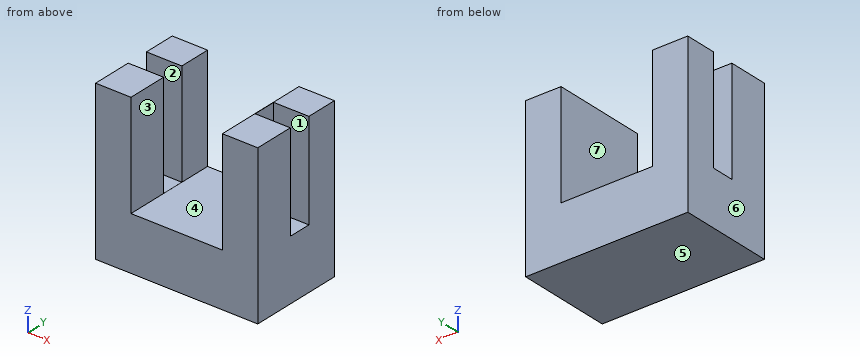
```python
from build123d import *

# Parameters (mm, degrees)
F1_DEPTH = 33.782
F2_DEPTH = 1.016
F3_W     = 12.5559801236
F3_H     = 8.0651557073
F4_DEPTH = 37.0078
F3_W_2   = 12.5338770449
F3_H_2   = 8.1778438762
F5_DEPTH = 34.544


with BuildPart() as f1:
    # F0 (on Front) → F1 (new body)
    with BuildSketch(Plane.XZ):
        Polygon((0, 56.0894832015), (0, 0), (56.5477348864, 0), (56.5477348864, 56.0894832015), (44.99989748, 56.0894832015), (44.99989748, 19.0630927682), (12.5559801236, 19.0630927682), (12.5559801236, 56.0894832015), align=None)
    extrude(amount=F1_DEPTH)

    # F2 (add): a face of the model
    f2_faces = [f1.faces().sort_by_distance(p)[0] for p in [
        (56.5477348864, -16.891, 28.0447416008),
    ]]
    extrude(f2_faces, amount=F2_DEPTH)

    # F3 (on face) → F4 (cut)
    with BuildSketch(Plane.XY.offset(56.0894832015)):
        with Locations((6.2779900618, -15.3971132822)):
            Rectangle(F3_W, F3_H)
    extrude(amount=-F4_DEPTH, mode=Mode.SUBTRACT)

    # F3 (on face) → F5 (cut)
    with BuildSketch(Plane.XY.offset(56.0894832015)):
        with Locations((6.2779900618, -15.3971132822)):
            Rectangle(F3_W, F3_H)
        with Locations((51.3402279466, -15.3407691978)):
            Rectangle(F3_W_2, F3_H_2)
    extrude(amount=-F5_DEPTH, mode=Mode.SUBTRACT)


solid = f1.part
```
Work out the finished part from the listing and answer in its coordinate system (mm). Face numbers are marked on the shaded views. A direction names the side the tool comes from. Coordinates: 2 decimals unless noted, no trailing zeros. Loops run counter-clockwise (first coordinate to the right, second up) from the corner with the lowest first, then second, coordinate; pieces in that order, holes last. Notation, with made-up numbers: M 84,38.5 L 110,38.5 A13 ccw 110,61.5 Z; hole C 50.25,-25.75 d4. An arc over 180 degrees is marked long. Use CSV: the item, a comma, the result in double quotes. Start each with the question number.
(1) Find section C-C, the plane x = 6. Give the vertices of the cut face in (y, z).
(2) Consider line 1 (Y direction, x = 5.5, z = 28.5); line 2 (X direction, y = -25, z = 51.5); line 3 (Z direction, x = 30, y = -14.5). Determine where each line is inside the solid, lowest interval first.
(3) Find section D-D, the plane y = -30.5. Give the vertices of the cut face in (x, z), then the cut area to 3 significant figures.
(4) For the marked faces 1, 2 and 3, determine the directions among +Z, -Z, +X, -X, +Y, -Y from which every point of the face is accessible in a straight line to the end or side of a thin tool.
(5) Given pin 1 Ø1.5 at (x, y) = (16.5, -15.5) entering from +Z; pin 2 Ø2.5 at (y, z) = (-15.5, 35) entering from +X, each flat-ended and moving along its own axis, determine where each tip first touches the part or whether it passes through.
(6) Find section B-B, the plane z = 34.5. Give the vertices of the cut face in (x, y), then the cut area to 3 significant figures.
(7) For a pull along X with two mould halves and no side action, classify the marked faces 4, 5, 6 and 7 as +X half, -X half, draft (parallel to the pull), parting line (faces both ways), or undercut.
Recorded:
1,outline,"M -33.78,0 L 0,0 L 0,56.09 L -11.36,56.09 L -11.36,19.08 L -19.43,19.08 L -19.43,56.09 L -33.78,56.09 Z"
2,line 1,"y = -33.78 to -19.43, -11.36 to 0"
2,line 2,"x = 0 to 12.56, 45 to 57.56"
2,line 3,"z = 0 to 19.06"
3,outline,"M 0,0 L 57.56,0 L 57.56,56.09 L 45,56.09 L 45,19.06 L 12.56,19.06 L 12.56,56.09 L 0,56.09 Z"
3,area,"2,030 mm^2"
4,face 1,"+Z, +X"
4,face 2,"+Z, -X"
4,face 3,"+Z, +Y, -Y"
5,pin 1,"stops at z = 19.06"
5,pin 2,"stops at x = 45.07"
6,outline,"M 0,-33.78 L 12.56,-33.78 L 12.56,-19.43 L 0,-19.43 Z; M 0,-11.36 L 12.56,-11.36 L 12.56,0 L 0,0 Z; M 45,-33.78 L 57.56,-33.78 L 57.56,-19.43 L 45.07,-19.43 L 45.07,-11.25 L 57.56,-11.25 L 57.56,0 L 45,0 Z"
6,area,"645 mm^2"
7,face 4,"undercut"
7,face 5,"draft"
7,face 6,"-X half"
7,face 7,"undercut"
